For this review, take the finished solid that the model builds, in its own axes (mm). A direction names the side the tool comes from. Give positions to 0.01 mm unless a question says otherwise; leave off trailing zeros. Loops run counter-clockwise (first coordinate to the right, second up) from the corner with the lowest first, then second, coordinate; pieces in that order, holes last.
```python
from build123d import *

# Parameters (mm, degrees)
BOSS_EXTRUDE1_DEPTH      = 12
BOSS_EXTRUDE1_DEPTH_BACK = 12
FILLET1_R                = 10
BOSS_EXTRUDE2_REACH      = 83.915
CUT_EXTRUDE1_DEPTH       = 98.519690427
CUT_EXTRUDE1_DEPTH_BACK  = 98.519690427
SKETCH5_R                = 13.665152344
CHAMFER1_SIZE            = 8
CHAMFER2_SIZE            = 1.6


with BuildPart() as part:
    # Sketch1 → Boss-Extrude1 (new, two sides: drawn at the far end of the back side and taken through both)
    with BuildSketch(Plane(origin=(0, 0, 0), x_dir=(1, 0, 0), z_dir=(0, 1, 0)).offset(-BOSS_EXTRUDE1_DEPTH_BACK)):
        with BuildLine():
            Line((-35, 0), (35, 0))
            ThreePointArc((35, 0), (46.17246087, -4.991197968), (49.909726541, -16.643184251))
            ThreePointArc((49.909726541, -16.643184251), (44.926099942, -43.406027638), (36.03300946, -69.135373954))
            ThreePointArc((36.03300946, -69.135373954), (31.487933236, -75.020695994), (24.674822271, -78))
            ThreePointArc((24.674822271, -78), (0, -80), (-24.674822271, -78))
            ThreePointArc((-24.674822271, -78), (-31.487933236, -75.020695994), (-36.03300946, -69.135373954))
            ThreePointArc((-36.03300946, -69.135373954), (-44.926099942, -43.406027638), (-49.909726541, -16.643184251))
            ThreePointArc((-49.909726541, -16.643184251), (-46.17246087, -4.991197968), (-35, 0))
        make_face()
    extrude(amount=BOSS_EXTRUDE1_DEPTH + BOSS_EXTRUDE1_DEPTH_BACK)

    # Fillet1
    fillet1_edges = [part.edges().sort_by_distance(p)[0] for p in [
        (-46.17246087, -12, 4.991197968),
        (-44.926099942, -12, 43.406027638),
        (-31.487933236, -12, 75.020695994),
        (46.17246087, 12, 4.991197968),
        (0, 12, 0),
        (-46.17246087, 12, 4.991197968),
        (-44.926099942, 12, 43.406027638),
        (-31.487933236, 12, 75.020695994),
        (0, -12, 80),
        (0, 12, 80),
        (31.487933236, 12, 75.020695994),
        (44.926099942, 12, 43.406027638),
        (31.487933236, -12, 75.020695994),
        (44.926099942, -12, 43.406027638),
        (46.17246087, -12, 4.991197968),
        (0, -12, 0),
    ]]
    fillet(fillet1_edges, radius=FILLET1_R)

    # Sketch2 → Revolve1 (revolve)
    with BuildSketch(Plane(origin=(0, 0, 0), x_dir=(1, 0, 0), z_dir=(0, 1, 0))):
        with BuildLine():
            Line((0, 0), (0, -55))
            ThreePointArc((0, -55), (17.465537495, -47.765537495), (24.7, -30.3))
            Line((24.7, -30.3), (24.7, 0))
            Line((24.7, 0), (0, 0))
        make_face()
    revolve(axis=Axis((0, 0, 0), (0, 0, 1)))

    # Sketch3 → Cut-Revolve1 (revolve, cut)
    with BuildSketch(Plane(origin=(0, 0, 0), x_dir=(1, 0, 0), z_dir=(0, 1, 0))):
        with BuildLine():
            Line((21.5, 0), (21.5, -30.3))
            ThreePointArc((21.5, -30.3), (15.202795796, -45.502795796), (0, -51.8))
            Line((0, -51.8), (0, 0))
            Line((0, 0), (21.5, 0))
        make_face()
    revolve(axis=Axis((0, 0, 0), (0, 0, 1)), mode=Mode.SUBTRACT)

    # Sketch4 → Boss-Extrude2 (add, up to next)
    with BuildSketch(Plane(origin=(0, 0, 20), x_dir=(-1, 0, 0), z_dir=(0, 0, -1)), mode=Mode.PRIVATE) as boss_extrude2_sk1:
        with BuildLine():
            Line((-16.099301227, 14.25), (16.099301227, 14.25))
            ThreePointArc((16.099301227, 14.25), (0, 21.5), (-16.099301227, 14.25))
        make_face()
    boss_extrude2_tool1 = extrude(boss_extrude2_sk1.sketch, amount=-BOSS_EXTRUDE2_REACH, mode=Mode.PRIVATE) - part.part
    # Sketch4 → Boss-Extrude2 (add, up to next)
    with BuildSketch(Plane(origin=(0, 0, 20), x_dir=(-1, 0, 0), z_dir=(0, 0, -1)), mode=Mode.PRIVATE) as boss_extrude2_sk2:
        with BuildLine():
            Line((-16.099301227, -14.25), (16.099301227, -14.25))
            ThreePointArc((16.099301227, -14.25), (0, -21.5), (-16.099301227, -14.25))
        make_face()
    boss_extrude2_tool2 = extrude(boss_extrude2_sk2.sketch, amount=-BOSS_EXTRUDE2_REACH, mode=Mode.PRIVATE) - part.part
    add(boss_extrude2_tool1.solids().sort_by_distance((0, 17.196475, 20))[0])
    add(boss_extrude2_tool2.solids().sort_by_distance((0, -17.196475, 20))[0])

    # Sketch5 → Cut-Extrude1 (cut, two sides: drawn at the far end of the back side and taken through both)
    with BuildSketch(Plane(origin=(0, 0, 0), x_dir=(1, 0, 0), z_dir=(0, 1, 0)).offset(-CUT_EXTRUDE1_DEPTH_BACK)):
        with Locations(Location((0, -61.334847656, 0), (0, 0, 322.861585756))):
            Circle(SKETCH5_R)
    extrude(amount=CUT_EXTRUDE1_DEPTH + CUT_EXTRUDE1_DEPTH_BACK, mode=Mode.SUBTRACT)

    # Chamfer1
    # the kernel refuses this chamfer: 8 mm, written as the material it takes off along each edge
    with BuildSketch(Plane(origin=(36.672765131, 14.25, 20), x_dir=(0, -0.02749587661058627, 0.9996219169112968), z_dir=(-1, 0, 0))) as chamfer1_piece_1_section:
        Polygon((CHAMFER1_SIZE * 0.999621916911, CHAMFER1_SIZE * 0.0274958766106), (-CHAMFER1_SIZE * 0.0274958766106, CHAMFER1_SIZE * 0.999621916911), (0, 0), align=None)
    chamfer1_piece_1 = extrude(amount=73.345530262, mode=Mode.PRIVATE)
    chamfer1_piece_1 = chamfer1_piece_1 & Plane(origin=(0, 0, 22.88602407), x_dir=(1, 0, 0), z_dir=(0, 0, 1)) * Cylinder(21.5, 179, mode=Mode.PRIVATE)
    add(chamfer1_piece_1, mode=Mode.SUBTRACT)
    with BuildSketch(Plane(origin=(36.672765131, -14.25, 20), x_dir=(0, 0.02749587661058627, 0.9996219169112968), z_dir=(-1, 0, 0))) as chamfer1_piece_2_section:
        Polygon((CHAMFER1_SIZE * 0.999621916911, -CHAMFER1_SIZE * 0.0274958766106), (-CHAMFER1_SIZE * 0.0274958766106, -CHAMFER1_SIZE * 0.999621916911), (0, 0), align=None)
    chamfer1_piece_2 = extrude(amount=73.345530262, mode=Mode.PRIVATE)
    chamfer1_piece_2 = chamfer1_piece_2 & Plane(origin=(0, 0, 22.88602407), x_dir=(1, 0, 0), z_dir=(0, 0, 1)) * Cylinder(21.5, 179, mode=Mode.PRIVATE)
    add(chamfer1_piece_2, mode=Mode.SUBTRACT)

    # Chamfer2
    chamfer2_edges = [part.edges().sort_by_distance(p)[0] for p in [
        (0, 24.7, 0),
        (0, -24.7, 0),
    ]]
    chamfer(chamfer2_edges, length=CHAMFER2_SIZE)


solid = part.part
```
Item 1: The part is to be moulded in two halves that separate along X. For faces 4 (the flat face through (0, -14.25, 35)), 5 (the flat face through (0.23, -17.02, 25.23)), 6 (the conical face through (0.486, 23.373, 0.278)), 7 (the cylindrical face through (-28.2, -8.99, 2.85)), say which applies: released by +X, released by -X, zero draft, split by the parting line, or undercut.
Answer:
face 4: undercut
face 5: undercut
face 6: split by the parting line
face 7: zero draft
Item 2: Clearance check with flat-ended pins moving along their axes: pin 1 Ø1.5 at (x, z) = (-11.5, 64) entering from +Y; pin 2 Ø10 at (x, z) = (36.5, 13) entering from -Y; pin 3 Ø2 at (y, z) = (-2, 47.5) entering from -X; pin 4 Ø20 at (x, z) = (-6.5, 39) entering from -Y (3 decimals). State where each tip first meets the part, or that it passes through.
Answer:
pin 1: passes through
pin 2: stops at y = -12
pin 3: stops at x = -44.08
pin 4: stops at y = -24.685
Item 3: Take a section at B-B on y = 0. Give the boundary of the cut face in (x, z).
Answer:
outline: (-49.91, 16.64) arc R15 ccw to (-35, 0) - (-21.5, 0) - (-21.5, 30.3) arc R21.5 cw to (-8, 50.26) arc R13.67 cw (long way) to (8, 50.26) arc R21.5 cw to (21.5, 30.3) - (21.5, 0) - (35, 0) arc R15 ccw to (49.91, 16.64) arc R183.27 ccw to (36.03, 69.14) arc R15 ccw to (24.67, 78) arc R153.21 ccw to (-24.67, 78) arc R15 ccw to (-36.03, 69.14) arc R183.27 ccw to start
Item 4: For L1, parallel to Y at x = 0, z = 20; L2, parallel to Y at x = -17, z = 21.5; L3, parallel to Y at x = -16.5, z = 60.5, list the stretches that pass through material, from the lowest coordinate up.
Answer:
L1: y = -24.7 to -21.5, 21.5 to 24.7
L2: y = -17.92 to -13.16, 13.16 to 17.92
L3: y = -12 to 12
Item 5: Take a section at A-A on x = 0. Give the boundary of the cut face in (y, z), and give its area (3 significant figures).
Answer:
outline: (-24.7, 1.6) - (-23.1, 0) - (-21.5, 0) - (-21.5, 20.75) - (-14.25, 28) - (-14.25, 46.4) arc R21.5 cw to (-12.67, 47.67) - (-17.56, 47.67) arc R24.7 ccw to (-24.7, 30.3) - close; (-10.66, 75) - (10.66, 75) arc R10 ccw to (2, 80) - (-2, 80) arc R10 ccw to start; (12.67, 47.67) arc R21.5 cw to (14.25, 46.4) - (14.25, 28) - (21.5, 20.75) - (21.5, 0) - (23.1, 0) - (24.7, 1.6) - (24.7, 30.3) arc R24.7 ccw to (17.56, 47.67) - close
area: 646 mm2
Item 6: Tool access review of faces 1 (the flat face through (-27, 12, 39)), 2 (the flat face through (28, -12, 39)), 3 (the flat face through (28, 12, 39)): name each direction out of +Z, -Z, +X, -X, +Y, -Y from which nothing blocks a thin tool from reaching the whole face with its end or side.
Answer:
face 1: +Z, -X, +Y
face 2: +Z, +X, -Y
face 3: +Z, +X, +Y
